Input: part model. Units: mm. Frame: model coordinates. Face numbers are marked on the shaded views. A direction names the side the tool comes from. Coordinates: 2 decimals unless noted, no trailing zeros. Order: outer loops, then holes, each group sorted by start corner. A loop starts at its lowest first (then second) coordinate and runs counter-clockwise, first axis right, second up.
from build123d import *

# Parameters (mm, degrees)
SKETCH2_W                      = 65.3415
SKETCH2_H                      = 177.8
BASE_FLANGE1_DEPTH             = 2.286
EDGE_FLANGE1_STRIP_W           = 19.304
EDGE_FLANGE1_STRIP_H           = 2.286
EDGE_FLANGE1_STRIP_CUT_DEPTH   = 177.8
EDGE_FLANGE1_STRIP_2_W         = 19.304
EDGE_FLANGE1_STRIP_2_H         = 2.286
EDGE_FLANGE1_STRIP_CUT_2_DEPTH = 177.8
EDGE_FLANGE1_DEPTH             = 177.8
EDGE_FLANGE1_BEND_DEPTH        = 177.8
CUT_EXTRUDE1_DEPTH             = 171.223828311
CUT_EXTRUDE1_DEPTH_BACK        = 171.223828311
CUT_EXTRUDE2_DEPTH             = 171.223828311
CUT_EXTRUDE2_DEPTH_BACK        = 171.223828311
SKETCH20_W                     = 141.560534952
SKETCH20_H                     = 182.926434851
EDGE_FLANGE3_STRIP_W           = 19.304
EDGE_FLANGE3_STRIP_H           = 2.286
EDGE_FLANGE3_STRIP_CUT_DEPTH   = 52
EDGE_FLANGE3_STRIP_2_W         = 19.304
EDGE_FLANGE3_STRIP_2_H         = 2.286
EDGE_FLANGE3_STRIP_CUT_2_DEPTH = 52
EDGE_FLANGE3_DEPTH             = 52
EDGE_FLANGE3_BEND_DEPTH        = 52
SKETCH30_R                     = 3.81
CUT_EXTRUDE3_DEPTH             = 129.336350021
SKETCH31_R                     = 4.3688
CUT_EXTRUDE4_DEPTH             = 129.336350021


# Sheet-metal steps are written as plain solids
with BuildPart() as part:
    # Sketch2 → Base-Flange1 (new body)
    with BuildSketch(Plane(origin=(0, 0, 0), x_dir=(1, 0, 0), z_dir=(0, 1, 0))):
        with Locations((2.25425, 63.5)):
            Rectangle(SKETCH2_W, SKETCH2_H)
    extrude(amount=-BASE_FLANGE1_DEPTH)

    # Edge-Flange1 strip (across the edge) → Edge-Flange1 strip cut (cut)
    with BuildSketch(Plane(origin=(-30.4165, 0, -152.4), x_dir=(1, 0, 0), z_dir=(0, 0, 1))):
        with Locations((-2.286, -1.143)):
            Rectangle(EDGE_FLANGE1_STRIP_W, EDGE_FLANGE1_STRIP_H)
    extrude(amount=EDGE_FLANGE1_STRIP_CUT_DEPTH, mode=Mode.SUBTRACT)

    # Edge-Flange1 strip 2 (across the edge) → Edge-Flange1 strip cut 2 (cut)
    with BuildSketch(Plane(origin=(34.925, 0, 25.4), x_dir=(-1, 0, 0), z_dir=(0, 0, -1))):
        with Locations((-2.286, -1.143)):
            Rectangle(EDGE_FLANGE1_STRIP_2_W, EDGE_FLANGE1_STRIP_2_H)
    extrude(amount=EDGE_FLANGE1_STRIP_CUT_2_DEPTH, mode=Mode.SUBTRACT)

    # Edge-Flange1 section (across the edge) → Edge-Flange1 (add)
    with BuildSketch(Plane(origin=(-30.4165, 0, -152.4), x_dir=(1, 0, 0), z_dir=(0, 0, 1))):
        with BuildLine():
            Line((0, 5.08), (0, 67.31))
            Line((0, 67.31), (2.286, 67.31))
            Line((2.286, 67.31), (2.286, 5.08))
            ThreePointArc((2.286, 5.08), (3.773897552, 1.487897552), (7.366, 0))
            Line((7.366, 0), (7.366, -2.286))
            ThreePointArc((7.366, -2.286), (2.15745145, -0.12854855), (0, 5.08))
        make_face()
    extrude(amount=EDGE_FLANGE1_DEPTH)

    # Edge-Flange1 section 2 (across the edge) → Edge-Flange1 bend (add)
    with BuildSketch(Plane(origin=(34.925, 0, 25.4), x_dir=(-1, 0, 0), z_dir=(0, 0, -1))):
        with BuildLine():
            Line((0, 5.08), (0, 67.31))
            Line((0, 67.31), (2.286, 67.31))
            Line((2.286, 67.31), (2.286, 5.08))
            ThreePointArc((2.286, 5.08), (3.773897552, 1.487897552), (7.366, 0))
            Line((7.366, 0), (7.366, -2.286))
            ThreePointArc((7.366, -2.286), (2.15745145, -0.12854855), (0, 5.08))
        make_face()
    extrude(amount=EDGE_FLANGE1_BEND_DEPTH)

    # Sketch19 → Cut-Extrude1 (cut, two sides: drawn at the far end of the back side and taken through both)
    with BuildSketch(Plane(origin=(0, 0, 0), x_dir=(0, 0, -1), z_dir=(1, 0, 0)).offset(-CUT_EXTRUDE1_DEPTH_BACK)):
        Polygon((-21.631039281, 5.08), (-21.631039281, -27.285513127), (-49.571039281, -27.285513127), (-49.571039281, 149.369143464), (35.341160719, 149.369143464), (35.341160719, 47.769143464), align=None)
    extrude(amount=CUT_EXTRUDE1_DEPTH + CUT_EXTRUDE1_DEPTH_BACK, mode=Mode.SUBTRACT)

    # Sketch20 → Cut-Extrude2 (cut, two sides: drawn at the far end of the back side and taken through both)
    with BuildSketch(Plane(origin=(0, 0, 0), x_dir=(0, 0, -1), z_dir=(1, 0, 0)).offset(-CUT_EXTRUDE2_DEPTH_BACK)):
        with Locations((158.121428195, 37.56832172)):
            Rectangle(SKETCH20_W, SKETCH20_H)
    extrude(amount=CUT_EXTRUDE2_DEPTH + CUT_EXTRUDE2_DEPTH_BACK, mode=Mode.SUBTRACT)

    # Edge-Flange3 strip (across the edge) → Edge-Flange3 strip cut (cut)
    with BuildSketch(Plane(origin=(-30.4165, 67.31, -35.341160719), x_dir=(0, -1, 0), z_dir=(0, 0, -1))):
        with Locations((-2.286, -1.143)):
            Rectangle(EDGE_FLANGE3_STRIP_W, EDGE_FLANGE3_STRIP_H)
    extrude(amount=EDGE_FLANGE3_STRIP_CUT_DEPTH, mode=Mode.SUBTRACT)

    # Edge-Flange3 strip 2 (across the edge) → Edge-Flange3 strip cut 2 (cut)
    with BuildSketch(Plane(origin=(34.925, 67.31, -87.341160719), x_dir=(0, -1, 0), z_dir=(0, 0, 1))):
        with Locations((-2.286, -1.143)):
            Rectangle(EDGE_FLANGE3_STRIP_2_W, EDGE_FLANGE3_STRIP_2_H)
    extrude(amount=EDGE_FLANGE3_STRIP_CUT_2_DEPTH, mode=Mode.SUBTRACT)

    # Edge-Flange3 section (across the edge) → Edge-Flange3 (add)
    with BuildSketch(Plane(origin=(-30.4165, 67.31, -35.341160719), x_dir=(0, -1, 0), z_dir=(0, 0, -1))):
        with BuildLine():
            Line((0, 5.08), (0, 30.734))
            Line((0, 30.734), (2.286, 30.734))
            Line((2.286, 30.734), (2.286, 5.08))
            ThreePointArc((2.286, 5.08), (3.773897552, 1.487897552), (7.366, 0))
            Line((7.366, 0), (7.366, -2.286))
            ThreePointArc((7.366, -2.286), (2.15745145, -0.12854855), (0, 5.08))
        make_face()
    extrude(amount=EDGE_FLANGE3_DEPTH)

    # Edge-Flange3 section 2 (across the edge) → Edge-Flange3 bend (add)
    with BuildSketch(Plane(origin=(34.925, 67.31, -87.341160719), x_dir=(0, -1, 0), z_dir=(0, 0, 1))):
        with BuildLine():
            Line((0, 5.08), (0, 30.734))
            Line((0, 30.734), (2.286, 30.734))
            Line((2.286, 30.734), (2.286, 5.08))
            ThreePointArc((2.286, 5.08), (3.773897552, 1.487897552), (7.366, 0))
            Line((7.366, 0), (7.366, -2.286))
            ThreePointArc((7.366, -2.286), (2.15745145, -0.12854855), (0, 5.08))
        make_face()
    extrude(amount=EDGE_FLANGE3_BEND_DEPTH)

    # Sketch30 → Cut-Extrude3 (cut, through all)
    with BuildSketch(Plane(origin=(0, 0, 0), x_dir=(1, 0, 0), z_dir=(0, 1, 0))):
        with Locations(Location((0, -10.995792601, 0), (0, 0, 270))):
            Circle(SKETCH30_R)
        with Locations(Location((0, 65.204207399, 0), (0, 0, 270))):
            Circle(SKETCH30_R)
    extrude(amount=-CUT_EXTRUDE3_DEPTH, mode=Mode.SUBTRACT)

    # Sketch31 → Cut-Extrude4 (cut, symmetric)
    with BuildSketch(Plane(origin=(0, 0, 0), x_dir=(1, 0, 0), z_dir=(0, 1, 0))):
        with Locations(Location((52.197, 73.441160719, 0), (0, 0, 270))):
            Circle(SKETCH31_R)
        with Locations(Location((52.197, 48.041160719, 0), (0, 0, 270))):
            Circle(SKETCH31_R)
    cut_extrude4 = extrude(amount=CUT_EXTRUDE4_DEPTH, both=True, mode=Mode.SUBTRACT)

    # Mirror1: Cut-Extrude4 across plane
    add(cut_extrude4.mirror(Plane(origin=(0, 0, 0), x_dir=(0, 0, 1), z_dir=(1, 0, 0))), mode=Mode.SUBTRACT)


solid = part.part
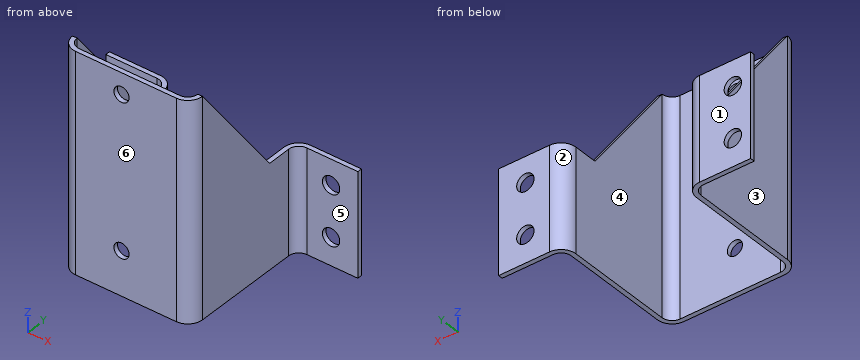
Item 1: Draft query along X for the marked faces 1, 2 and 3. Return one class per face: pulls with the +X half, pulls with the -X half, needs draft (parallel to the pull), parting line crosses it, or undercut.
Response values:
face 1: needs draft
face 2: undercut
face 3: pulls with the -X half
Item 2: Cut plane B-B on y = 50. Return loops of the section in (x, z) (1 decimal), then the cut area to 3 significant figures.
Response values:
outline: (-30.4, -87.3) - (-28.1, -87.3) - (-28.1, -35.3) - (-30.4, -35.3) - close; (32.6, -87.3) - (34.9, -87.3) - (34.9, -35.3) - (32.6, -35.3) - close
area: 238 mm2
Item 3: Ray query, probe 1 along X at (y, z) = (27, -24) (1 decimal); probe 2 along Y at (x, z) = (-2, -37); probe 3 along Y at (x, z) = (30.5, -9.5). Return the intervals inside material, ascending.
Response values:
probe 1: x = -30.4 to -28.1, 32.6 to 34.9
probe 2: y = -2.29 to 0
probe 3: y = -1.67 to 0.94
Item 4: Cut plane C-C on z = -55.5. Return loops of the section in (x, y) (1 decimal).
Response values:
outline: (-61.2, 65) - (-35.5, 65) arc R5.1 cw to (-30.4, 59.9) - (-30.4, 5.1) arc R7.4 ccw to (-23.1, -2.3) - (27.6, -2.3) arc R7.4 ccw to (34.9, 5.1) - (34.9, 59.9) arc R5.1 cw to (40, 65) - (65.7, 65) - (65.7, 67.3) - (40, 67.3) arc R7.4 ccw to (32.6, 59.9) - (32.6, 5.1) arc R5.1 cw to (27.6, 0) - (-23.1, 0) arc R5.1 cw to (-28.1, 5.1) - (-28.1, 59.9) arc R7.4 ccw to (-35.5, 67.3) - (-61.2, 67.3) - close
Item 5: Cut plane D-D on z = -72.5. Return loops of the section in (x, y) (1 decimal), then the cut area to 3 significant figures.
Response values:
outline: (-61.2, 65) - (-56.5, 65) - (-56.5, 67.3) - (-61.2, 67.3) - close; (-47.9, 65) - (-35.5, 65) arc R5.1 cw to (-30.4, 59.9) - (-30.4, 5.1) arc R7.4 ccw to (-23.1, -2.3) - (27.6, -2.3) arc R7.4 ccw to (34.9, 5.1) - (34.9, 59.9) arc R5.1 cw to (40, 65) - (47.9, 65) - (47.9, 67.3) - (40, 67.3) arc R7.4 ccw to (32.6, 59.9) - (32.6, 5.1) arc R5.1 cw to (27.6, 0) - (-23.1, 0) arc R5.1 cw to (-28.1, 5.1) - (-28.1, 59.9) arc R7.4 ccw to (-35.5, 67.3) - (-47.9, 67.3) - close; (56.5, 65) - (65.7, 65) - (65.7, 67.3) - (56.5, 67.3) - close
area: 534 mm2
Item 6: Cut plane A-A on x = 0. Return loops of the section in (y, z), then the cut area to 3 significant figures.
Response values:
outline: (-2.29, -87.34) - (0, -87.34) - (0, -69.01) - (-2.29, -69.01) - close; (-2.29, -61.39) - (0, -61.39) - (0, 7.19) - (-2.29, 7.19) - close; (-2.29, 14.81) - (0, 14.81) - (0, 21.63) - (-2.29, 21.63) - close
area: 214 mm2
Item 7: Access query for the marked faces 4, 5 and 6. Directions: +Z, -Z, +X, -X, +Y, -Y. A direction counts if a zero-diameter tool reaches every point of the face in a straight line with its end or side. Return the directions, or none.
Response values:
face 4: +Z, -Z, +Y
face 5: +Z, -Z, +X, -Y
face 6: +Z, -Z, +X, -X, -Y
Item 8: Pin query (flat end, axial travel): pin 1 Ø6 at (x, z) = (-28.5, -3.5) entering from -Y; pin 2 Ø15 at (x, z) = (7, -53.5) entering from +Y; pin 3 Ø15.5 at (x, y) = (-51.5, 58) entering from +Z; pin 4 Ø14 at (x, z) = (-52.2, -48.04) entering from +Y. Return the tip coordinate at first contact, or that it passes through.
Response values:
pin 1: stops at y = -1.87
pin 2: stops at y = 0
pin 3: stops at z = -35.34
pin 4: stops at y = 67.31
